Source: CAD feature listing. Evaluate the final solid. Frame: model axes, mm. Face numbers are marked on the shaded views. A direction names the side the tool comes from. Round coordinates to 2 decimals unless told otherwise and drop trailing zeros. Write each loop counter-clockwise with the first axis right and the second up, starting at its lowest first coordinate (ties: lowest second). Pieces come first, ordered by that corner, then holes. Notation, with made-up numbers: M 50,48.25 L 72,48.25 A12 cw 72,65.25 Z; hole C 26.25,12 d11. An arc over 180 degrees is marked long. Answer in a Markdown table with one row per item.
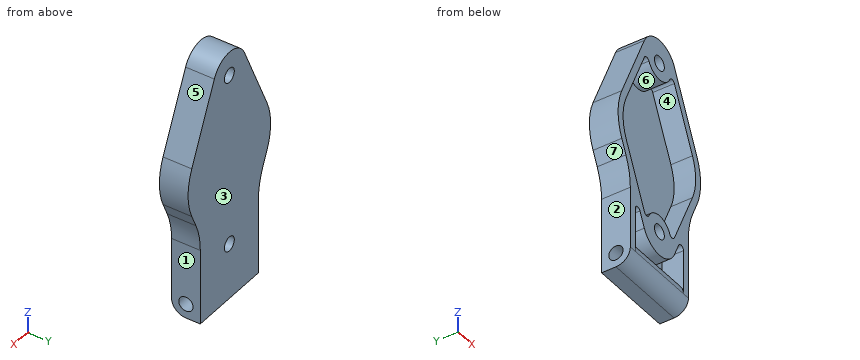
from build123d import *

# Parameters (mm, degrees)
F0_R     = 2
F1_DEPTH = 8
F2_DEPTH = 2
F3_R     = 20
F4_R     = 1
F6_D     = 4
F7_R     = 3.99999


# Not quite as in the source:
# - a fillet or chamfer is up to 0.001 mm smaller than in the source, because OpenCascade refuses the exact size
# - a feature names something its author has since deleted; it is built from what else it names


with BuildPart() as f1:
    # F0 (on Front) → F1 (new body)
    with BuildSketch(Plane.XZ):
        with BuildLine():
            Line((15.1970139668, 6.8636525628), (6.0880650012, 27.0320429916))
            ThreePointArc((6.0880650012, 27.0320429916), (0, 30.9626), (-6.0880650012, 27.0320429916))
            Line((-6.0880650012, 27.0320429916), (-15.1970139668, 6.8636525628))
            ThreePointArc((-15.1970139668, 6.8636525628), (-16.6751, 0), (-15.1970139668, -6.8636525628))
            Line((-15.1970139668, -6.8636525628), (-11.75, -14.4957870449))
            Line((-11.75, -14.4957870449), (-9.75, -18.9240455641))
            Line((-9.75, -18.9240455641), (-6.0880650012, -27.0320429916))
            ThreePointArc((-6.0880650012, -27.0320429916), (0, -30.9626), (6.0880650012, -27.0320429916))
            Line((6.0880650012, -27.0320429916), (9.75, -18.9240455641))
            Line((9.75, -18.9240455641), (11.75, -14.4957870449))
            Line((11.75, -14.4957870449), (15.1970139668, -6.8636525628))
            ThreePointArc((15.1970139668, -6.8636525628), (16.6751, 0), (15.1970139668, 6.8636525628))
        make_face()
        with Locations((0, -24.2824)):
            Circle(F0_R, mode=Mode.SUBTRACT)
        with BuildLine():
            Line((-13.3742945868, 6.0404308054), (-6.0462846285, 22.2655920687))
            ThreePointArc((-6.0462846285, 22.2655920687), (-5.1436901116, 22.8539427752), (-4.2309206889, 22.2815046593))
            ThreePointArc((-4.2309206889, 22.2815046593), (0, 19.6022), (4.2309206889, 22.2815046593))
            ThreePointArc((4.2309206889, 22.2815046593), (5.1436901116, 22.8539427752), (6.0462846285, 22.2655920687))
            Line((6.0462846285, 22.2655920687), (13.3742945868, 6.0404308054))
            ThreePointArc((13.3742945868, 6.0404308054), (14.6751, 0), (13.3742945868, -6.0404308054))
            Line((13.3742945868, -6.0404308054), (6.0462846285, -22.2655920687))
            ThreePointArc((6.0462846285, -22.2655920687), (5.1436901116, -22.8539427752), (4.2309206889, -22.2815046593))
            ThreePointArc((4.2309206889, -22.2815046593), (0, -19.6022), (-4.2309206889, -22.2815046593))
            ThreePointArc((-4.2309206889, -22.2815046593), (-5.1436901116, -22.8539427752), (-6.0462846285, -22.2655920687))
            Line((-6.0462846285, -22.2655920687), (-13.3742945868, -6.0404308054))
            ThreePointArc((-13.3742945868, -6.0404308054), (-14.6751, 0), (-13.3742945868, 6.0404308054))
        make_face(mode=Mode.SUBTRACT)
        with Locations((0, 24.2824)):
            Circle(F0_R, mode=Mode.SUBTRACT)
        Polygon((11.75, -40), (11.75, -14.4957870449), (9.75, -18.9240455641), (9.75, -32), (-9.75, -32), (-9.75, -18.9240455641), (-11.75, -14.4957870449), (-11.75, -40), align=None)
    extrude(amount=F1_DEPTH)

    # F0 (on Front) → F2 (join)
    with BuildSketch(Plane.XZ):
        with BuildLine():
            ThreePointArc((-4.2309206889, 22.2815046593), (-5.1436901116, 22.8539427752), (-6.0462846285, 22.2655920687))
            Line((-6.0462846285, 22.2655920687), (-13.3742945868, 6.0404308054))
            ThreePointArc((-13.3742945868, 6.0404308054), (-14.6751, 0), (-13.3742945868, -6.0404308054))
            Line((-13.3742945868, -6.0404308054), (-6.0462846285, -22.2655920687))
            ThreePointArc((-6.0462846285, -22.2655920687), (-5.1436901116, -22.8539427752), (-4.2309206889, -22.2815046593))
            ThreePointArc((-4.2309206889, -22.2815046593), (0, -19.6022), (4.2309206889, -22.2815046593))
            ThreePointArc((4.2309206889, -22.2815046593), (5.1436901116, -22.8539427752), (6.0462846285, -22.2655920687))
            Line((6.0462846285, -22.2655920687), (13.3742945868, -6.0404308054))
            ThreePointArc((13.3742945868, -6.0404308054), (14.6751, 0), (13.3742945868, 6.0404308054))
            Line((13.3742945868, 6.0404308054), (6.0462846285, 22.2655920687))
            ThreePointArc((6.0462846285, 22.2655920687), (5.1436901116, 22.8539427752), (4.2309206889, 22.2815046593))
            ThreePointArc((4.2309206889, 22.2815046593), (0, 19.6022), (-4.2309206889, 22.2815046593))
        make_face()
        with BuildLine():
            Line((9.75, -32), (9.75, -18.9240455641))
            Line((9.75, -18.9240455641), (6.0880650012, -27.0320429916))
            ThreePointArc((6.0880650012, -27.0320429916), (0, -30.9626), (-6.0880650012, -27.0320429916))
            Line((-6.0880650012, -27.0320429916), (-9.75, -18.9240455641))
            Line((-9.75, -18.9240455641), (-9.75, -32))
            Line((-9.75, -32), (9.75, -32))
        make_face()
    extrude(amount=F2_DEPTH)

    # F3
    f3_edges = [f1.edges().sort_by_distance(p)[0] for p in [
        (11.75, -4, -14.495787),
        (-11.75, -4, -14.495787),
    ]]
    fillet(f3_edges, radius=F3_R)

    # F4
    f4_edges = [f1.edges().sort_by_distance(p)[0] for p in [
        (9.75, -5, -18.924046),
        (-9.75, -5, -18.924046),
    ]]
    fillet(f4_edges, radius=F4_R)

    # F6 (through all)
    with Locations(Plane.YZ.offset(11.75)):
        with Locations((-4, -36)):
            Hole(F6_D / 2)

    # F7 (radius 4 in the source; OpenCascade refuses exactly that, so slightly less here)
    f7_edges = [f1.edges().sort_by_distance(p)[0] for p in [
        (0, -8, -40),
        (0, -8, -32),
    ]]
    fillet(f7_edges, radius=F7_R)


solid = f1.part
Q1. Material intervals for probe 1 along Z at (x, y) = (-3.25, -4); probe 2 along Z at (x, y) = (6.5, -4); probe 3 along X at (y, z) = (-6.5, -26.5), sorted ascending.
Solutions:
| item | result |
|---|---|
| probe 1 | z = -40 to -38, -34 to -32, -30.12 to -20.91, 20.91 to 30.12 |
| probe 2 | z = -40 to -38, -34 to -32, -26.12 to -21.26, 21.26 to 26.12 |
| probe 3 | x = -11.75 to -9.75, -6.33 to 6.33, 9.75 to 11.75 |
Q2. Access query for the marked faces 1, 2, 3 and 4. Directions: +Z, -Z, +X, -X, +Y, -Y. A direction counts if a zero-diameter tool reaches every point of the face in a straight line with its end or side. Return the directions, or none.
Solutions:
| item | result |
|---|---|
| face 1 | -Z, +X, +Y, -Y |
| face 2 | -Z, -X, +Y, -Y |
| face 3 | +Z, -Z, +X, -X, +Y |
| face 4 | -Y |
Q3. Section B-B (x = 11). Return loops of the section in (y, z), and give its area (3 significant figures).
Solutions:
| item | result |
|---|---|
| outline | M -8,-36 A4 ccw -4,-40 L 0,-40 L 0,16.16 L -8,16.16 L -8,11.3 L -2,11.3 L -2,-11.3 L -8,-11.3 Z; hole C -4,-36 d4 |
| area | 298 mm2 |
Q4. Contact query for flat-ended pins moving along their axis: pin 1 Ø3 at (y, z) = (-4, 4) entering from +X; pin 2 Ø4 at (y, z) = (-2, -30) entering from -X; pin 3 Ø3 at (x, y) = (10, -4.5) entering from +Z; pin 4 Ø3 at (x, z) = (0, 24.28) entering from -Y. Output: stop coordinate, or through.
Solutions:
| item | result |
|---|---|
| pin 1 | stops at x = 16.49 |
| pin 2 | stops at x = -11.75 |
| pin 3 | stops at z = 21.69 |
| pin 4 | passes through |
Q5. Section C-C (z = -1). Return loops of the section in (x, y).
Solutions:
| item | result |
|---|---|
| outline | M -16.65,-8 L -14.64,-8 L -14.64,-2 L 14.64,-2 L 14.64,-8 L 16.65,-8 L 16.65,0 L -16.65,0 Z |
Q6. Section D-D (y = -0.75). Return loops of the section in (x, z).
Solutions:
| item | result |
|---|---|
| outline | M -15.2,-6.86 L -13.52,-10.57 A20 cw -11.75,-18.8 L -11.75,-40 L 11.75,-40 L 11.75,-18.8 A20 cw 13.52,-10.57 L 15.2,-6.86 A16.68 ccw 15.2,6.86 L 6.09,27.03 A6.68 ccw -6.09,27.03 L -15.2,6.86 A16.68 ccw Z; hole C 0,-24.28 d4; hole C 0,24.28 d4 |
Q7. Section A-A (x = 1). State how many separate pieces and enclosed holes the cut face has, and give its area (3 significant figures).
Solutions:
| item | result |
|---|---|
| separate pieces | 3 |
| enclosed holes | 1 |
| area | 249 mm2 |
Q8. Pull-direction query (X, two-part tool) for the marked faces 5, 6 and 7; classes: pulls with the +X half, pulls with the -X half, needs draft (parallel to the pull), parting line crosses it, or undercut.
Solutions:
| item | result |
|---|---|
| face 5 | pulls with the +X half |
| face 6 | undercut |
| face 7 | pulls with the -X half |
